The listing builds one solid part. Answer for the finished solid, in the listing's coordinates (mm). A direction names the side the tool comes from. Coordinates: 2 decimals unless noted, no trailing zeros. Loops run counter-clockwise (first coordinate to the right, second up) from the corner with the lowest first, then second, coordinate; pieces in that order, holes last. Notation, with made-up numbers: (81.5, -15) - (134.5, -15) arc R29 ccw to (134.5, 24) - close; hole circle Ø7 at (1, -13.5). An arc over 180 degrees is marked (long way). Put each result on its own line as item: value.
```python
from build123d import *

# Parameters (mm, degrees)
SKETCH1_W                  = 15
SKETCH1_H                  = 10
BOSS_EXTRUDE1_DEPTH        = 75
SKETCH2_R                  = 3
CUT_EXTRUDE1_DEPTH         = 4.5
SKETCH3_R                  = 1.75
CUT_EXTRUDE2_DEPTH         = 76.574466588
CHAMFER1_SIZE              = 0.5
LPATTERN1_COUNT            = 4
LPATTERN1_PITCH            = 40
CHAMFER1_OF_LPATTERN1_SIZE = 0.5
CHAMFER2_SIZE              = 0.5


with BuildPart() as part:
    # Sketch1 → Boss-Extrude1 (new, symmetric)
    with BuildSketch(Plane.XY):
        Rectangle(SKETCH1_W, SKETCH1_H)
    extrude(amount=BOSS_EXTRUDE1_DEPTH, both=True)

    # Sketch2 → Cut-Extrude1 (cut)
    with BuildSketch(Plane(origin=(0, 5, 0), x_dir=(1, 0, 0), z_dir=(0, 1, 0))):
        with Locations(Location((0, -60, 0), (0, 0, 180))):
            Circle(SKETCH2_R)
    cut_extrude1 = extrude(amount=-CUT_EXTRUDE1_DEPTH, mode=Mode.SUBTRACT)

    # Sketch3 → Cut-Extrude2 (cut, through all)
    with BuildSketch(Plane(origin=(0, 0.5, 0), x_dir=(1, 0, 0), z_dir=(0, 1, 0))):
        with Locations(Location((0, -60, 0), (0, 0, 180))):
            Circle(SKETCH3_R)
    cut_extrude2 = extrude(amount=-CUT_EXTRUDE2_DEPTH, mode=Mode.SUBTRACT)

    # Chamfer1
    chamfer1_edges = [part.edges().sort_by_distance(p)[0] for p in [
        (3, 5, 60),
        (1.75, -5, 60),
    ]]
    chamfer(chamfer1_edges, length=CHAMFER1_SIZE)

    # LPattern1: Cut-Extrude1, Cut-Extrude2 ×4
    with Locations(*[(0, 0, -i * LPATTERN1_PITCH) for i in range(1, LPATTERN1_COUNT)]):
        add(cut_extrude1, mode=Mode.SUBTRACT)
        add(cut_extrude2, mode=Mode.SUBTRACT)

    # Chamfer1 of LPattern1
    chamfer1_of_lpattern1_edges = [part.edges().sort_by_distance(p)[0] for p in [
        (3, 5, 20),
        (1.75, -5, 20),
        (3, 5, -20),
        (1.75, -5, -20),
        (3, 5, -60),
        (1.75, -5, -60),
    ]]
    chamfer(chamfer1_of_lpattern1_edges, length=CHAMFER1_OF_LPATTERN1_SIZE)

    # Chamfer2
    chamfer2_edges = [part.edges().sort_by_distance(p)[0] for p in [
        (-7.5, 5, 0),
        (7.5, 5, 0),
        (7.5, -5, 0),
        (-7.5, -5, 0),
    ]]
    chamfer(chamfer2_edges, length=CHAMFER2_SIZE)


solid = part.part
```
1) The part is cut by section A-A (z = 20). Give the vertices of the cut face in (x, y), and give its area (3 significant figures).
Found:
outline: (-7.5, -4.5) - (-7, -5) - (-2.25, -5) - (-1.75, -4.5) - (-1.75, 0.5) - (-3, 0.5) - (-3, 4.5) - (-3.5, 5) - (-7, 5) - (-7.5, 4.5) - close; (1.75, -4.5) - (2.25, -5) - (7, -5) - (7.5, -4.5) - (7.5, 4.5) - (7, 5) - (3.5, 5) - (3, 4.5) - (3, 0.5) - (1.75, 0.5) - close
area: 103 mm^2
2) For a pull along X with two mould halves and no side action, classify faces 3 (the face through (7.5, 0, 1)), 4 (the face through (0.65, 2.53, 17.07)), 5 (the face through (0, 0, -75)) as pulls with the +X half, pulls with the -X half, needs draft (parallel to the pull), parting line crosses it, or undercut.
Found:
face 3: pulls with the +X half
face 4: undercut
face 5: needs draft
3) The part is cut by section B-B (y = -1). Give the vertices of the cut face in (x, z), and give its area (3 significant figures).
Found:
outline: (-7.5, -75) - (7.5, -75) - (7.5, 75) - (-7.5, 75) - close; hole circle Ø3.5 at (0, -60); hole circle Ø3.5 at (0, -20); hole circle Ø3.5 at (0, 20); hole circle Ø3.5 at (0, 60)
area: 2,210 mm^2
4) The part is cut by section C-C (x = 0). State how many separate pieces and enclosed holes the cut face has, and give its area (3 significant figures).
Found:
separate pieces: 5
enclosed holes: 0
area: 1,310 mm^2
5) This flat-tipped pin is pushed along its axis until it touches: pin 1 (5.5 mm diameter, centred on x = 0, z = 20, fed in from +Y). Where does it stop, or does it pass through?
Found:
pin 1: stops at y = 0.5
6) For faces 1 (the face through (0.38, -1.96, -61.71)), 2 (the face through (0, 3, 63)), determine the directions among +Z, -Z, +X, -X, +Y, -Y from which every point of the face is accessible in a straight line to the end or side of a thin tool.
Found:
face 1: +Y, -Y
face 2: +Y
7) Straight lines are drawn through the part: L1, parallel to Z at x = 0, y = 3.75; L2, parallel to Z at x = 0, y = -2.2; L3, parallel to Y at x = 2.75, z = -60.5. For each, find the intervals that lie inside material, in ascending order. Write a range as [from, to].
Found:
L1: z = [-75, -63], [-57, -23], [-17, 17], [23, 57], [63, 75]
L2: z = [-75, -61.75], [-58.25, -21.75], [-18.25, 18.25], [21.75, 58.25], [61.75, 75]
L3: y = [-5, 0.5]
